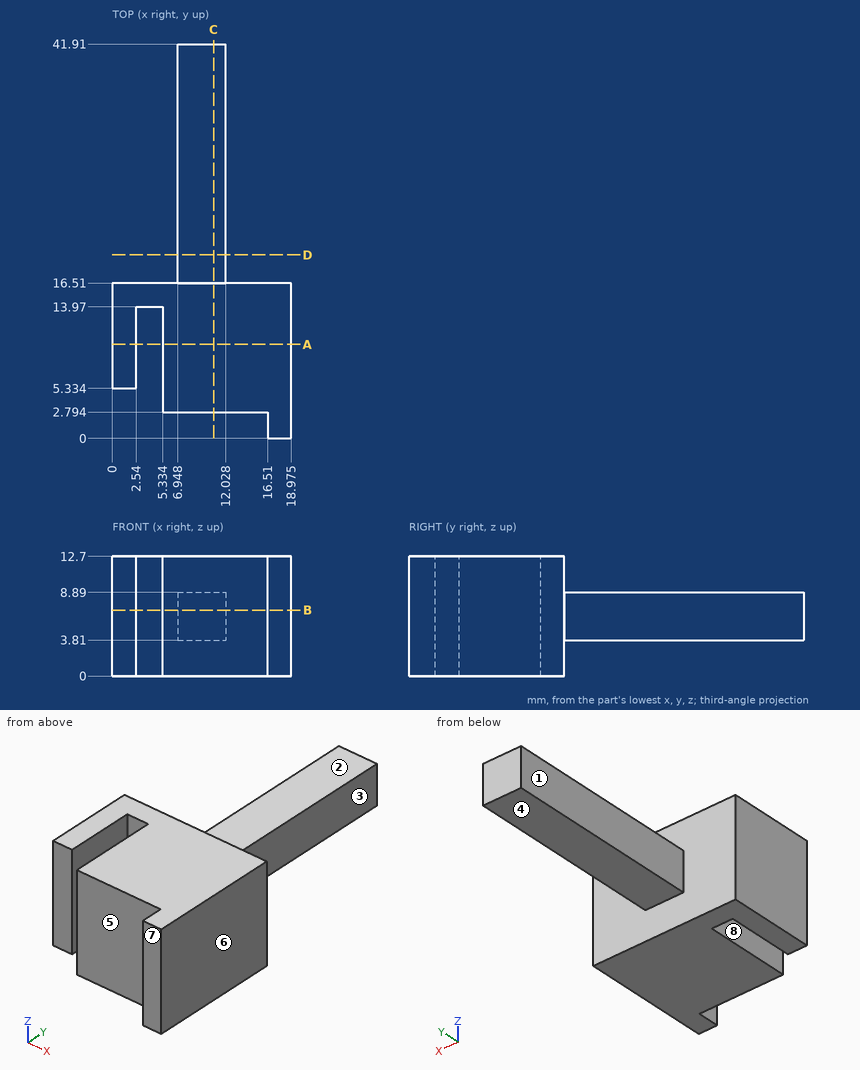
Design review of the part shown in the three views and the two pictorial views. Dimensions are in mm from the part's minimum x, y and z. A direction names the side the tool comes from. Coordinates: 2 decimals unless noted, no trailing zeros. Order: outer loops, then holes, each group sorted by start corner. A loop starts at its lowest first (then second) coordinate and runs counter-clockwise, first axis right, second up.
1) Take a section at D-D, the plane y = 19.5. Give the boundary of the cut face in (x, z).
2) For the marked faces 1, 2, 3, 4 and 5, list the 3-axis set-ups (+Z, -Z, +X, -X, +Y, -Y) from which the entire face can be reached by the end or side of a thin tool; tool diameter is ignored.
3) Clearance check with flat-ended pins moving along their axes: pin 1 (3 mm diameter, centred on x = 11.5, y = 25.5, fed in from -Z); pin 2 (5.5 mm diameter, centred on y = 28.5, z = 6, fed in from -X); pin 3 (4 mm diameter, centred on x = 10, y = 23.5, fed in from +Z). State where each tip first meets the part, or that it passes through.
4) Mouldability with a two-part tool opening along X and no side actions: class the marked faces 6, 7 and 8 as +X half, -X half, draft (parallel to the pull), parting line (faces both ways), or undercut.
5) Take a section at A-A, the plane y = 10. Give the boundary of the cut face in (x, z) (1 decimal).
6) Take a section at C-C, the plane x = 10.75. Give the boundary of the cut face in (y, z).
7) Take a section at B-B, the plane z = 7. Give the boundary of the cut face in (x, y) (1 decimal).
8) Wall thickness on line 1 along X through (y, z) = (12.5, 8.75) (1 decimal); line 2 along Y through (x, z) = (9.75, 10.5); line 3 along Z through (x, y) = (11.75, 27): over which ranges is each line inside the solid? List them lowest first.
Returned:
1. outline: (6.95, 3.81) - (12.03, 3.81) - (12.03, 8.89) - (6.95, 8.89) - close
2. face 1: +Z, -Z, -X, +Y
2. face 2: +Z, +X, -X, +Y
2. face 3: +Z, -Z, +X, +Y
2. face 4: -Z, +X, -X, +Y
2. face 5: +Z, -Z, -X, -Y
3. pin 1: stops at z = 3.81
3. pin 2: stops at x = 6.95
3. pin 3: stops at z = 8.89
4. face 6: +X half
4. face 7: draft
4. face 8: undercut
5. outline: (0, 0) - (2.5, 0) - (2.5, 12.7) - (0, 12.7) - close; (5.3, 0) - (19, 0) - (19, 12.7) - (5.3, 12.7) - close
6. outline: (2.79, 0) - (16.51, 0) - (16.51, 3.81) - (41.91, 3.81) - (41.91, 8.89) - (16.51, 8.89) - (16.51, 12.7) - (2.79, 12.7) - close
7. outline: (0, 5.3) - (2.5, 5.3) - (2.5, 14) - (5.3, 14) - (5.3, 2.8) - (16.5, 2.8) - (16.5, 0) - (19, 0) - (19, 16.5) - (12, 16.5) - (12, 41.9) - (6.9, 41.9) - (6.9, 16.5) - (0, 16.5) - close
8. line 1: x = 0 to 2.5, 5.3 to 19
8. line 2: y = 2.79 to 16.51
8. line 3: z = 3.81 to 8.89
